CAD build for the part. Positions are in the model's coordinates, mm. Face numbers are marked on the shaded views. A direction names the side the tool comes from. Round coordinates to 2 decimals unless told otherwise and drop trailing zeros. Loops run counter-clockwise (first coordinate to the right, second up) from the corner with the lowest first, then second, coordinate; pieces in that order, holes last. Notation, with made-up numbers: (-18.5, -14) -> (34.5, -14) arc R19 cw to (34.5, 22) -> close; hole circle Ø4 at (9.25, 22). An arc over 180 degrees is marked (long way). Answer as CSV lines item,"result".
```python
from build123d import *

# Parameters (mm, degrees)
F0_R         = 25
F1_DEPTH     = 53
F2_R         = 26
F3_DEPTH     = 10
F4_R         = 22.8291590373
F5_DEPTH     = 3
F6_R         = 21.5
F7_DEPTH     = 2
F8_R         = 18.5
F9_DEPTH     = 5
F10_R        = 21.5
F11_DEPTH    = 2
F12_R        = 20
F13_DEPTH    = 2
F14_R        = 18.5
F15_DEPTH    = 2
F16_R        = 25
F17_DEPTH    = 35
F18_R        = 20
F19_DEPTH    = 32
F20_S5_R     = 18.5
F20_T6_DEPTH = 37
F22_R        = 5
F25_DEPTH    = 52.3
F26_T1_DEPTH = 15.5791600382
F26_T3_DEPTH = 15.5791600382
F27_R        = 14.5
F28_DEPTH    = 128


# Not quite as in the source:
# - a fillet or chamfer that OpenCascade refuses, or shapes differently, is made with other operations: its cross-section is extruded or revolved along the edge and cut away or added


with BuildPart() as f1:
    # F0 (on Front) → F1 (new body)
    with BuildSketch(Plane.XZ):
        Circle(F0_R)
    extrude(amount=F1_DEPTH)

    # F2 (on face) → F3 (join)
    with BuildSketch(Plane(origin=(0, 0, 0), x_dir=(-1, 0, 0), z_dir=(0, 1, 0))):
        Circle(F2_R)
    extrude(amount=F3_DEPTH)

    # F4 (on face) → F5 (join)
    with BuildSketch(Plane.XZ.offset(53)):
        Circle(F4_R)
    extrude(amount=F5_DEPTH)

    # F6 (on face) → F7 (join)
    with BuildSketch(Plane.XZ.offset(56)):
        Circle(F6_R)
    extrude(amount=F7_DEPTH)

    # F8 (on face) → F9 (join)
    with BuildSketch(Plane.XZ.offset(58)):
        Circle(F8_R)
    extrude(amount=F9_DEPTH)

    # F10 (on face) → F11 (join)
    with BuildSketch(Plane.XZ.offset(63)):
        Circle(F10_R)
    extrude(amount=F11_DEPTH)

    # F12 (on face) → F13 (join)
    with BuildSketch(Plane.XZ.offset(65)):
        Circle(F12_R)
    extrude(amount=F13_DEPTH)

    # F14 (on face) → F15 (join)
    with BuildSketch(Plane.XZ.offset(67)):
        Circle(F14_R)
    extrude(amount=F15_DEPTH)

    # F16 (on face) → F17 (join)
    with BuildSketch(Plane.XZ.offset(69)):
        Circle(F16_R)
    extrude(amount=F17_DEPTH)

    # F18 (on face) → F19 (cut)
    with BuildSketch(Plane.XZ.offset(104)):
        Circle(F18_R)
    extrude(amount=-F19_DEPTH, mode=Mode.SUBTRACT)

    # F20: chamfer of 7 on 1 edges, made by hand


with BuildPart() as f20_tool2:
    # F20_s3 → F20_t4 (revolve)
    with BuildSketch(Plane.XY):
        Polygon((25, -76), (18, -69), (25, -69), align=None)
    revolve(axis=Axis((0, -69, 0), (0, -1, 0)))

    # F20_s5 → F20_t6 (cut, symmetric)
    with BuildSketch(Plane.XZ.offset(72.5)):
        Circle(F20_S5_R)
    extrude(amount=F20_T6_DEPTH, both=True, mode=Mode.SUBTRACT)


with BuildPart() as f1_1:
    add(f1.part)

    # F20_t1: cut F20_tool2
    add(f20_tool2.part, mode=Mode.SUBTRACT)

    # F21: chamfer of 3 x 30 on 1 edges, made by hand

    # F21_s1 → F21_t2 (revolve, cut)
    with BuildSketch(Plane.XY):
        Polygon((25, -74), (22, -104), (25, -104), align=None)
    revolve(axis=Axis((0, -104, 0), (0, -1, 0)), mode=Mode.SUBTRACT)

    # F22
    f22_edges = [f1_1.edges().sort_by_distance(p)[0] for p in [
        (-24.818182, -75.818182, 0),
    ]]
    fillet(f22_edges, radius=F22_R)

    # F24 (on offset) → F25 (cut)
    with BuildSketch(Plane.YZ.offset(26.9)):
        with BuildLine():
            Line((-78, -31.0485586524), (-78, -28.3997934312))
            add(Edge.make_bspline(
                [(-78, -28.3997934312), (-98.6184179783, -3.1667915173), (-82.4469923973, 1.2942913454), (-107.4011772871, 17.0474909246)],
                knots=[0, 0, 0, 0, 54.1284110351, 54.1284110351, 54.1284110351, 54.1284110351], degree=3))
            Line((-107.4011772871, 17.0474909246), (-107.4011772871, -31.0485586524))
            Line((-107.4011772871, -31.0485586524), (-78, -31.0485586524))
        make_face()
    extrude(amount=-F25_DEPTH, mode=Mode.SUBTRACT)

    # F26: fillet of radius 5 on 2 edges, made by hand

    # F26_s2 → F26_t1 (cut)
    with BuildSketch(Plane.YZ.offset(7.0799043749)):
        with BuildLine():
            ThreePointArc((-102.0117387885, 13.3536507945), (-103.4757188766, 15.1160616448), (-104.0004, 17.346317106))
            Line((-104.0004, 17.346317106), (-104.50064, 17.346317106))
            ThreePointArc((-104.50064, 17.346317106), (-104.50024, 16.0708587935), (-104.50024, 14.795400481))
            Line((-104.50024, 14.795400481), (-104.286297169, 14.3851883546))
            ThreePointArc((-104.286297169, 14.3851883546), (-103.2925012303, 13.6788063197), (-102.3131126673, 12.9543841634))
            Line((-102.3131126673, 12.9543841634), (-102.0117387885, 13.3536507945))
        make_face()
    extrude(amount=F26_T1_DEPTH, mode=Mode.SUBTRACT)

    # F26_s4 → F26_t3 (cut)
    with BuildSketch(Plane.YZ.offset(-22.6590644131)):
        with BuildLine():
            ThreePointArc((-102.0117387885, 13.3536507945), (-103.4757188766, 15.1160616448), (-104.0004, 17.346317106))
            Line((-104.0004, 17.346317106), (-104.50064, 17.346317106))
            ThreePointArc((-104.50064, 17.346317106), (-104.50024, 16.0708587935), (-104.50024, 14.795400481))
            Line((-104.50024, 14.795400481), (-104.286297169, 14.3851883546))
            ThreePointArc((-104.286297169, 14.3851883546), (-103.2925012303, 13.6788063197), (-102.3131126673, 12.9543841634))
            Line((-102.3131126673, 12.9543841634), (-102.0117387885, 13.3536507945))
        make_face()
    extrude(amount=F26_T3_DEPTH, mode=Mode.SUBTRACT)

    # F27 (on face) → F28 (cut)
    with BuildSketch(Plane(origin=(0, 10, 0), x_dir=(-1, 0, 0), z_dir=(0, 1, 0))):
        Circle(F27_R)
    extrude(amount=-F28_DEPTH, mode=Mode.SUBTRACT)


solid = f1_1.part
```
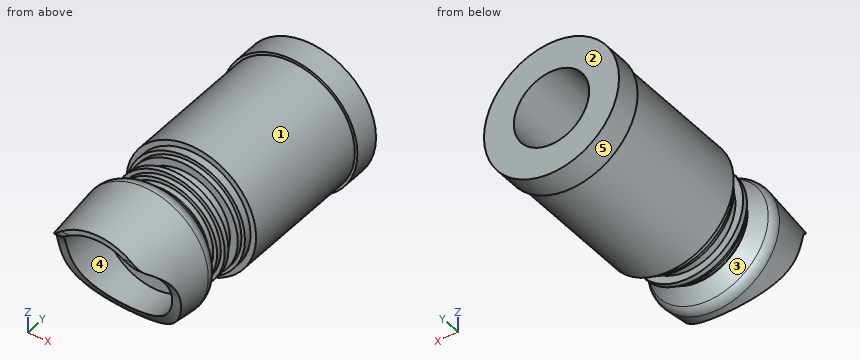
Q1. Slice it at A-A, the plane y = -45. Give the cut face in (x, z), and give its area (3 significant figures).
Results:
outline,"circle Ø50 at (0, 0); hole circle Ø29 at (0, 0)"
area,"1,300 mm2"
Q2. Drop flat-ended pins along their axis: pin 1 Ø6 at (x, y) = (-3, -83) entering from -Z; pin 2 Ø2 at (x, z) = (-5, -19) entering from -Y; pin 3 Ø6 at (x, z) = (-18.5, -4.5) entering from -Y. Give the stop position or say it passes through.
Results:
pin 1,"z = -24.31"
pin 2,"y = -84.62"
pin 3,"y = -91.15"
Q3. Two-plate mould, pull along Y, no slides. Class the marked faces 1, 2 and 3: pulls with the +Y half, pulls with the -Y half, needs draft (parallel to the pull), parting line crosses it, or undercut.
Results:
face 1,"needs draft"
face 2,"pulls with the +Y half"
face 3,"undercut"
Q4. Probe L1, parallel to Y at x = 19.5, z = -0.5; L2, parallel to Z at x = 0, y = -32.5; L3, parallel to X at y = -88, z = 0. List the from-to ranges inside material, lowest first. Write a range as [from, to].
Results:
L1,"[-72, -70.51], [-67, -63], [-58, 10]"
L2,"[-25, -14.5], [14.5, 25]"
L3,"[-23.6, -20], [20, 23.6]"
Q5. Tool access for the marked faces 4 and 5: list every direction of +Z, -Z, +X, -X, +Y, -Y with a clear straight run to the whole face (end or side of a thin tool).
Results:
face 4,"-Y"
face 5,"+Y, -Y"
